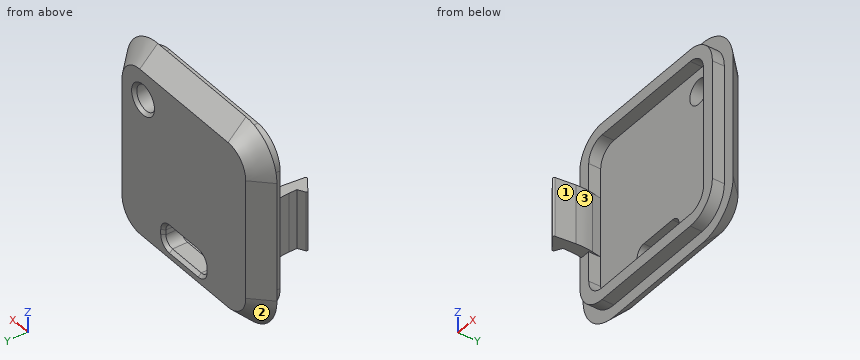
from build123d import *

# Parameters (mm, degrees)
CROQUIS1_W              = 34
CROQUIS1_H              = 34
SALIENTE_EXTRUIR1_DEPTH = 3
REDONDEO1_R             = 7
CHAFL_N1_SIZE           = 3
CROQUIS2_R              = 2.087433524
CROQUIS2_W              = 9.5
CROQUIS2_H              = 3.8
CORTAR_EXTRUIR1_DEPTH   = 25.228082879
REDONDEO2_R             = 1.5
CHAFL_N2_SIZE           = 0.5
SALIENTE_EXTRUIR2_DEPTH = 5
REDONDEO3_R             = 0.2
REDONDEO4_R             = 0.2
REDONDEO5_R             = 10
SALIENTE_EXTRUIR3_DEPTH = 2


with BuildPart() as part:
    # Croquis1 → Saliente-Extruir1 (new body)
    with BuildSketch(Plane(origin=(0, 0, 0), x_dir=(1, 0, 0), z_dir=(0, 1, 0))):
        Rectangle(CROQUIS1_W, CROQUIS1_H)
    extrude(amount=SALIENTE_EXTRUIR1_DEPTH)

    # Redondeo1
    redondeo1_edges = [part.edges().sort_by_distance(p)[0] for p in [
        (17, 1.5, 17),
        (-17, 1.5, 17),
        (-17, 1.5, -17),
        (17, 1.5, -17),
    ]]
    fillet(redondeo1_edges, radius=REDONDEO1_R)

    # Chaflán1
    chafl_n1_edges = [part.edges().sort_by_distance(p)[0] for p in [
        (17, 3, 0),
        (14.949747468, 3, -14.949747468),
        (14.949747468, 3, 14.949747468),
        (0, 3, -17),
        (0, 3, 17),
        (-14.949747468, 3, -14.949747468),
        (-14.949747468, 3, 14.949747468),
        (-17, 3, 0),
    ]]
    chamfer(chafl_n1_edges, length=CHAFL_N1_SIZE - 0.0001)  # a hair under: the kernel refuses the full size

    # Croquis2 → Cortar-Extruir1 (cut, through all)
    with BuildSketch(Plane(origin=(0, 3, 0), x_dir=(1, 0, 0), z_dir=(0, 1, 0))):
        with Locations(Location((9.259969099, -9.25223211, 0), (0, 0, 270))):
            Circle(CROQUIS2_R)
        with Locations((0, 10.712955835)):
            Rectangle(CROQUIS2_W, CROQUIS2_H)
    extrude(amount=-CORTAR_EXTRUIR1_DEPTH, mode=Mode.SUBTRACT)

    # Redondeo2
    redondeo2_edges = [part.edges().sort_by_distance(p)[0] for p in [
        (4.75, 1.5, -12.612955835),
        (4.75, 1.5, -8.812955835),
        (-4.75, 1.5, -8.812955835),
        (-4.75, 1.5, -12.612955835),
    ]]
    fillet(redondeo2_edges, radius=REDONDEO2_R)

    # Chaflán2
    chafl_n2_edges = [part.edges().sort_by_distance(p)[0] for p in [
        (9.259969099, 3, 7.164798586),
        (0, 3, -8.812955835),
        (-4.75, 3, -10.712955835),
        (4.75, 3, -10.712955835),
        (0, 3, -12.612955835),
        (-4.310660172, 3, -9.252295663),
        (4.310660172, 3, -9.252295663),
        (4.310660172, 3, -12.173616007),
        (-4.310660172, 3, -12.173616007),
    ]]
    chamfer(chafl_n2_edges, length=CHAFL_N2_SIZE)

    # Croquis3 → Saliente-Extruir2 (add, symmetric)
    with BuildSketch(Plane.XY):
        Polygon((-15.871019058, -6.008290377), (-14.471019058, -5.2), (-14.471019058, -3), (-15, 0), (-13, 0), (-12.471019058, -3), (-13, -8), align=None)
    extrude(amount=SALIENTE_EXTRUIR2_DEPTH, both=True)

    # Redondeo3
    redondeo3_edges = [part.edges().sort_by_distance(p)[0] for p in [
        (-13, -8, 0),
    ]]
    fillet(redondeo3_edges, radius=REDONDEO3_R)

    # Redondeo4
    redondeo4_edges = [part.edges().sort_by_distance(p)[0] for p in [
        (-15.871019058, -6.008290377, 0),
    ]]
    fillet(redondeo4_edges, radius=REDONDEO4_R)

    # Redondeo5
    redondeo5_edges = [part.edges().sort_by_distance(p)[0] for p in [
        (-14.471019058, -3, 0),
        (-12.471019058, -3, 0),
    ]]
    fillet(redondeo5_edges, radius=REDONDEO5_R)

    # Croquis4 → Saliente-Extruir3 (add)
    with BuildSketch(Plane.XZ):
        with BuildLine():
            Line((-10, 15), (10, 15))
            ThreePointArc((10, 15), (13.535533906, 13.535533906), (15, 10))
            Line((15, 10), (15, -10))
            ThreePointArc((15, -10), (13.535533906, -13.535533906), (10, -15))
            Line((10, -15), (-10, -15))
            ThreePointArc((-10, -15), (-13.535533906, -13.535533906), (-15, -10))
            Line((-15, -10), (-15, 10))
            ThreePointArc((-15, 10), (-13.535533906, 13.535533906), (-10, 15))
        make_face()
        with BuildLine():
            Line((-13, 10), (-13, -10))
            ThreePointArc((-13, -10), (-12.121320344, -12.121320344), (-10, -13))
            Line((-10, -13), (10, -13))
            ThreePointArc((10, -13), (12.121320344, -12.121320344), (13, -10))
            Line((13, -10), (13, 10))
            ThreePointArc((13, 10), (12.121320344, 12.121320344), (10, 13))
            Line((10, 13), (-10, 13))
            ThreePointArc((-10, 13), (-12.121320344, 12.121320344), (-13, 10))
        make_face(mode=Mode.SUBTRACT)
    extrude(amount=SALIENTE_EXTRUIR3_DEPTH)


solid = part.part
Work out the finished part from the listing and answer in its coordinate system (mm). Face numbers are marked on the shaded views. Round coordinates to 2 decimals unless told otherwise and drop trailing zeros. Order: outer loops, then holes, each group sorted by start corner. A loop starts at its lowest first (then second) coordinate and runs counter-clockwise, first axis right, second up. Notation, with made-up numbers: M 29.5,65 L 85.5,65 A21 ccw 85.5,92 Z; hole C 60.25,-25 d4. An arc over 180 degrees is marked long. One line per item, written item: value.
Q1. Find section C-C on y = -1. Write down the section's boundary in (x, z), then the cut area to 3 significant figures.
Derived:
outline: M -15,-10 A5 ccw -10,-15 L 10,-15 A5 ccw 15,-10 L 15,10 A5 ccw 10,15 L -10,15 A5 ccw -15,10 Z; hole M -13,-10 A3 ccw -10,-13 L 10,-13 A3 ccw 13,-10 L 13,10 A3 ccw 10,13 L -10,13 A3 ccw -13,10 L -13,5 L -12.82,5 L -12.82,-5 L -13,-5 Z
area: 212 mm²
Q2. Straight lines are drawn through the part: line 1 (Y direction, x = -9, z = -5); line 2 (Y direction, x = -5.5, z = 14); line 3 (X direction, y = -1.75, z = -6.5). For each, find the intervals that lie inside material, in ascending order.
Derived:
line 1: 0 to 3
line 2: -2 to 3
line 3: -15 to -13, 13 to 15
Q3. Flat-ended cylindrical pins translate along their axes: pin 1 (1.5 mm diameter, centred on y = 1.5, z = -8, fed in from +X); pin 2 (2 mm diameter, centred on y = 2, z = -6, fed in from +X); pin 3 (6 mm diameter, centred on x = 13, z = 2.5, fed in from -Y); pin 4 (12 mm diameter, centred on x = -8.5, z = 7.5, fed in from -Y). Find the tip coordinate at first contact, or state that the pin passes through.
Derived:
pin 1: x = 16.25
pin 2: x = 16
pin 3: y = -2
pin 4: y = -7.84
Q4. Determine the mould class of the marked faces 1, 2 and 3 for opening direction Y: released by +Y, released by -Y, zero draft, split by the parting line, or undercut.
Derived:
face 1: released by -Y
face 2: released by +Y
face 3: undercut
